Source: three-view drawing plus pictorial views. Frame: mm from the lowest corner of the part. A direction names the side the tool comes from. Coordinates: 2 decimals unless noted, no trailing zeros. Write each loop counter-clockwise with the first axis right and the second up, starting at its lowest first coordinate (ties: lowest second). Pieces come first, ordered by that corner, then holes. Notation, with made-up numbers: (14.25, -12) - (24.25, -12) arc R26 cw to (24.25, 16) - close; hole circle Ø5 at (58.5, 58). An arc over 180 degrees is marked (long way). Put each result on its own line as item: value.
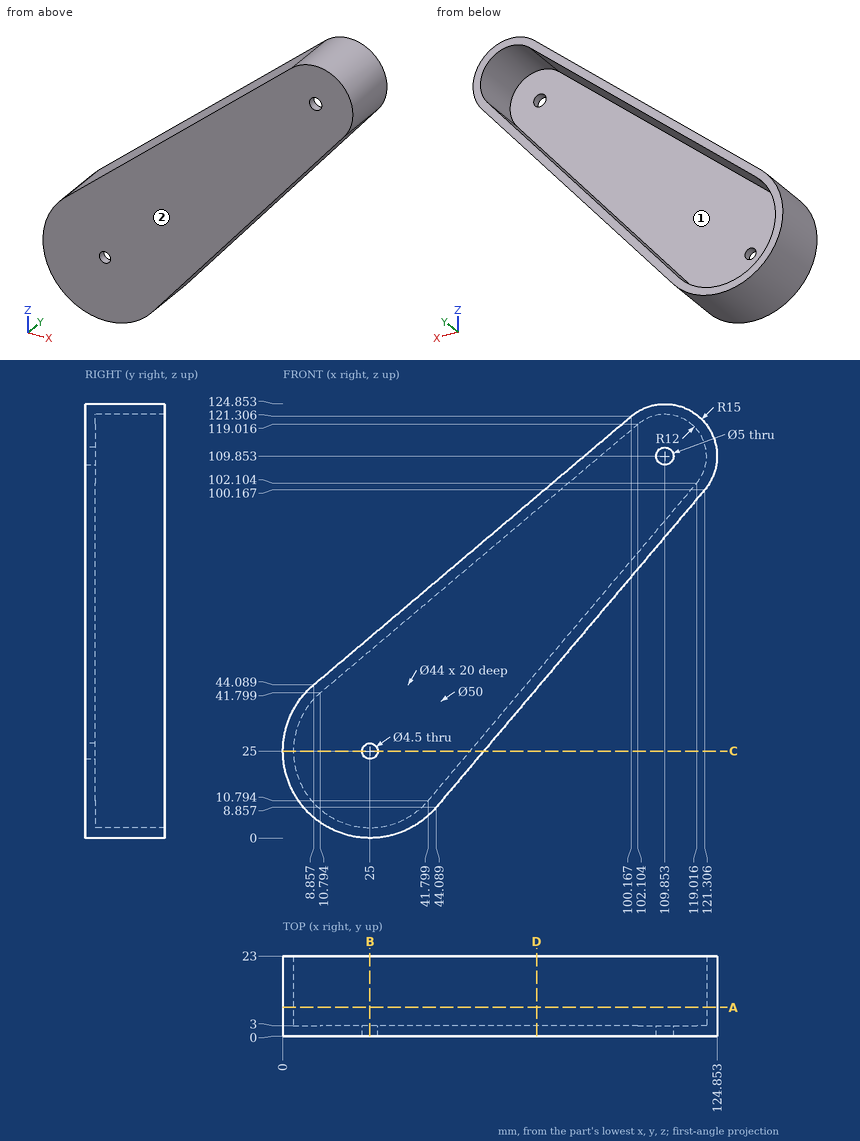
1. Section query D-D (x = 73). Return loops of the section in (y, z).
Answer below:
outline: (0, 43.04) - (23, 43.04) - (23, 47.69) - (3, 47.69) - (3, 94.4) - (23, 94.4) - (23, 98.33) - (0, 98.33) - close
2. Section query A-A (y = 8.25). Return loops of the section in (x, z) (1 decimal), then the cut area to 3 significant figures.
Answer below:
outline: (8.9, 44.1) arc R25 ccw (long way) to (44.1, 8.9) - (121.3, 100.2) arc R15 ccw to (100.2, 121.3) - close; hole (10.8, 41.8) arc R22 ccw (long way) to (41.8, 10.8) - (119, 102.1) arc R12 ccw to (102.1, 119) - close
area: 1,070 mm²
3. Pin query (flat end, axial travel): pin 1 Ø4 at (y, z) = (5.5, 63.5) entering from +X; pin 2 Ø8 at (y, z) = (3, 85) entering from +X; pin 3 Ø4 at (y, z) = (20.5, 98) entering from -X. Return the tip coordinate at first contact, or that it passes through.
Answer below:
pin 1: stops at x = 91.99
pin 2: stops at x = 111.86
pin 3: stops at x = 70.24
4. Set-up query: the marked faces 1 and 2. Return all of +Z, -Z, +X, -X, +Y, -Y with unobstructed straight access to the full face (end or side cutting, diameter ignored); none if empty.
Answer below:
face 1: +Y
face 2: +Z, -Z, +X, -X, -Y
5. Section query C-C (z = 25). Return loops of the section in (x, y), then the cut area to 3 significant figures.
Answer below:
outline: (0, 0) - (22.75, 0) - (22.75, 3) - (3, 3) - (3, 23) - (0, 23) - close; (27.25, 0) - (57.74, 0) - (57.74, 23) - (53.81, 23) - (53.81, 3) - (27.25, 3) - close
area: 298 mm²
6. Ray query, probe 1 along Y at (x, z) = (74, 74.5); probe 2 along X at (y, z) = (19.75, 89) (1 decimal); probe 3 along Z at (x, y) = (23, 20.75). Return the intervals inside material, ascending. Write a range as from..to.
Answer below:
probe 1: y = 0..3
probe 2: x = 62..66.6, 107.9..111.9
probe 3: z = 0.08..3.09, 52.12..56.05
7. Section query B-B (x = 25). Return loops of the section in (y, z).
Answer below:
outline: (0, 0) - (23, 0) - (23, 3) - (3, 3) - (3, 22.75) - (0, 22.75) - close; (0, 27.25) - (3, 27.25) - (3, 53.81) - (23, 53.81) - (23, 57.74) - (0, 57.74) - close
